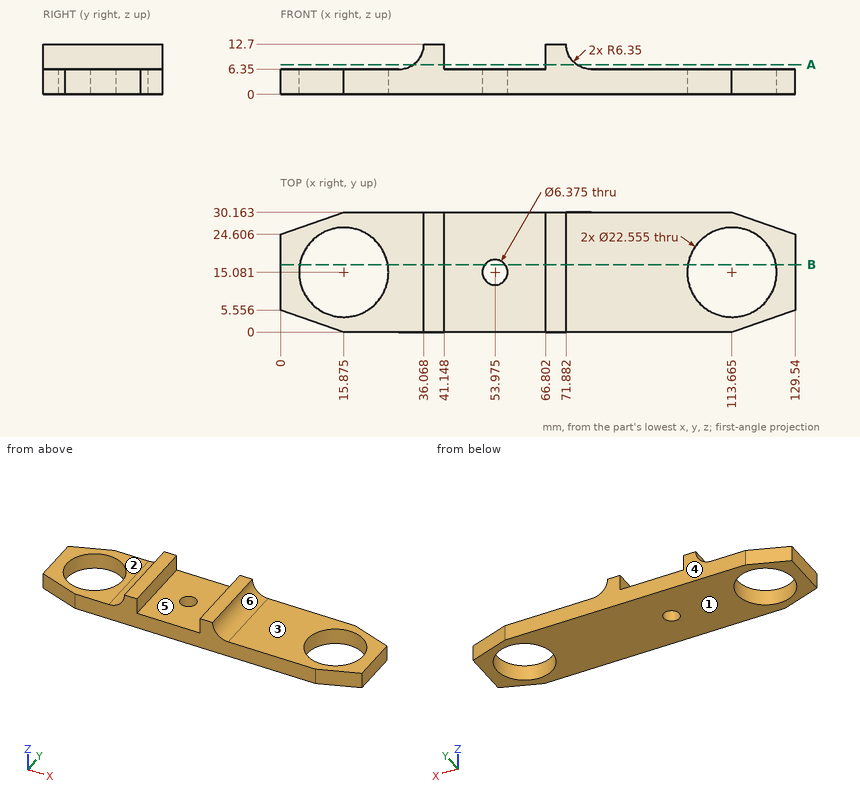
Here's the drawing with two shaded views (mm, measured from the low corner). I have some questions. A direction names the side the tool comes from. Coordinates: 2 decimals unless noted, no trailing zeros. Loops run counter-clockwise (first coordinate to the right, second up) from the corner with the lowest first, then second, coordinate; pieces in that order, holes last. Notation, with made-up numbers: (-7.75, 85.5) - (37.25, 85.5) arc R19 cw to (37.25, 118.5) - close; hole circle Ø4 at (49, 28). An arc over 180 degrees is marked (long way). Answer as CSV lines item,"result". Start each with the question number.
1) Suppose I cut it at A-A (z = 7.5). Please give me the cut outline in (x, y).
2) Thinking about a two-plate mould opening in X: for the marked faces 4, 5 and 6, which applies, pulls with the +X half, pulls with the -X half, needs draft (parallel to the pull), parting line crosses it, or undercut?
3) I need wall thicknesses on line 1 (X direction, y = 22, z = 2.5); line 2 (X direction, y = 8, z = 3.75); line 3 (X direction, y = 13, z = 1.25). Which ranges of each line are inside material? Lowest first, please. Write a range as from..to.
4) Which directions (+Z, -Z, +X, -X, +Y, -Y) give clear straight access to the entire face, cutting with the end or side of a thin tool? Please do the marked faces 1, 2 and 3.
5) Suppose I cut it at B-B (y = 17). Count the separate pieces of the cut face and the enclosed holes in it, plus the area to 3 significant figures.
6) For pin 1 (4 mm diameter, centred on x = 31, y = 11.5, fed in from +Z) (1 decimal); pin 2 (1.9 mm diameter, centred on y = 15, z = 10, fed in from +X) (1 decimal); pin 3 (1.9 mm diameter, centred on y = 8.5, z = 11, fed in from -X), each with a flat end and sliding along its axis, tell me the tip position at first contact or that it passes through.
Check result:
1,outline,"(33.36, 0) - (41.15, 0) - (41.15, 30.16) - (33.36, 30.16) - close; (66.8, 0) - (74.59, 0) - (74.59, 30.16) - (66.8, 30.16) - close"
2,face 4,"needs draft"
2,face 5,"undercut"
2,face 6,"pulls with the +X half"
3,line 1,"x = 0..6.97, 24.78..104.76, 122.57..129.54"
3,line 2,"x = 0..7.1, 24.65..104.89, 122.44..129.54"
3,line 3,"x = 0..4.79, 26.96..51.56, 56.39..102.58, 124.75..129.54"
4,face 1,"-Z, +X, -X, +Y, -Y"
4,face 2,"+Z, -X, +Y, -Y"
4,face 3,"+Z, +X, +Y, -Y"
5,separate pieces,"4"
5,enclosed holes,"0"
5,area,"590 mm²"
6,pin 1,"stops at z = 7.3"
6,pin 2,"stops at x = 73"
6,pin 3,"stops at x = 35.49"
